The listing builds one solid part. Answer for the finished solid, in the listing's coordinates (mm). Coordinates: 2 decimals unless noted, no trailing zeros. Order: outer loops, then holes, each group sorted by start corner. A loop starts at its lowest first (then second) coordinate and runs counter-clockwise, first axis right, second up.
```python
from build123d import *

# Parameters (mm, degrees)
F1_DEPTH = 12.7
F3_D     = 12.7
F5_D     = 6.35
F7_D     = 6.35
F9_D     = 6.35
F11_D    = 6.35


with BuildPart() as f1:
    # F0 (on Front) → F1 (new body)
    with BuildSketch(Plane.XZ):
        with BuildLine():
            Line((-326.100796, -8.113854), (-326.100796, -204.056984))
            Line((-326.100796, -204.056984), (4.099204, -204.056984))
            Line((4.099204, -204.056984), (4.099204, -80.450462))
            ThreePointArc((4.099204, -80.450462), (18.97818, -44.529437), (54.899204, -29.650462))
            Line((54.899204, -29.650462), (181.899204, -29.650462))
            ThreePointArc((181.899204, -29.650462), (253.438217, -76.024305), (266.565871, 8.213623))
            ThreePointArc((266.565871, 8.213623), (241.514438, 42.546778), (232.699367, 84.123628))
            Line((232.699367, 84.123628), (119.216243, 164.528722))
            ThreePointArc((119.216243, 164.528722), (77.53434, 181.786259), (32.489865, 179.296508))
            Line((32.489865, 179.296508), (-326.100796, -8.113854))
        make_face()
    extrude(amount=F1_DEPTH)

    # F3 (through all)
    with Locations(Plane.XZ.offset(12.7)):
        with Locations((232.699204, -29.650462), (-268.950796, -191.356984)):
            Hole(F3_D / 2)

    # F5 (through all)
    with Locations(Plane.XZ.offset(12.7)):
        with Locations((-319.750796, -89.756984)):
            Hole(F5_D / 2)

    # F7 (through all)
    with Locations(Plane.XZ.offset(12.7)):
        with Locations((-2.250796, -89.756984)):
            Hole(F7_D / 2)

    # F9 (through all)
    with Locations(Plane.XZ.offset(12.7)):
        with Locations((35.026812, 168.661091)):
            Hole(F9_D / 2)

    # F11 (through all)
    with Locations(Plane.XZ.offset(12.7)):
        with Locations((-278.057724, 0)):
            Hole(F11_D / 2)


solid = f1.part
```
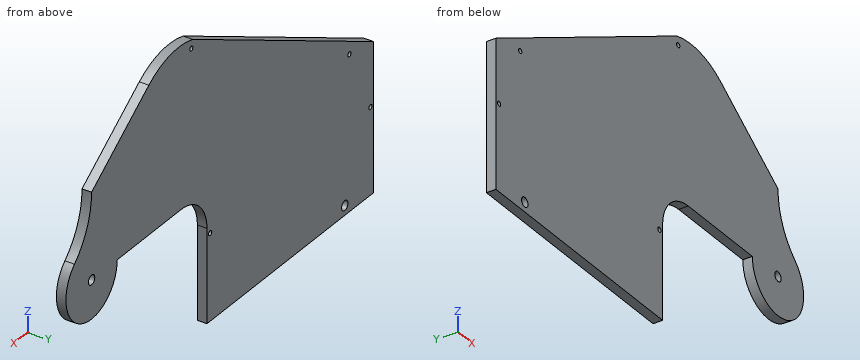
1) A cutting plane is placed at C-C, the plane z = -106.5. Write down the section's boundary in (x, y), plus the area to 3 significant figures.
2) A cutting plane is placed at B-B, the plane y = -7.5. Count the separate pieces of the cut face and the enclosed holes in it, plus the area to 3 significant figures.
3) A cutting plane is placed at A-A, the plane z = -47.5. Write down the section's boundary in (x, y), plus the area to 3 significant figures.
4) A cutting plane is placed at D-D, the plane x = -36. Write down the section's boundary in (y, z), plus the area to 3 significant figures.
5) Straight lines are drawn through the part: probe 1 along X at (y, z) = (-11, 167); probe 2 along X at (y, z) = (-3, -116); probe 3 along Z at (x, y) = (-5, -4.25). For each, find the intervals that lie inside material, in ascending order.
6) Each of these flat-tipped pins is pushed along its axis until it touches: P1, Ø4, axis at x = 97, y = -8.5, coming from the -Z side; P2, Ø4, axis at x = 219.5, y = -8, coming from the +Z side; P3, Ø6, axis at y = -7, z = 87.5, coming from the +X side; P4, Ø5, axis at x = -2.25, z = -89.76, coming from the -Y side. Where does it stop, or does it pass through?
Working result:
1. outline: (-326.1, -12.7) - (4.1, -12.7) - (4.1, 0) - (-326.1, 0) - close
1. area: 4,190 mm2
2. separate pieces: 1
2. enclosed holes: 6
2. area: 141,000 mm2
3. outline: (-326.1, -12.7) - (16.24, -12.7) - (16.24, 0) - (-326.1, 0) - close; (185.14, -12.7) - (280.26, -12.7) - (280.26, 0) - (185.14, 0) - close
3. area: 5,560 mm2
4. outline: (-12.7, -204.06) - (0, -204.06) - (0, 143.5) - (-12.7, 143.5) - close
4. area: 4,410 mm2
5. probe 1: x = 8.96 to 32.32, 37.73 to 115.56
5. probe 2: x = -326.1 to 4.1
5. probe 3: z = -204.06 to -91.35, -88.17 to 159.7
6. P1: stops at z = -29.65
6. P2: stops at z = 94.89
6. P3: stops at x = 232.17
6. P4: passes through
